Autodesk Inventor part; units mm, degrees
ref_plane "YZ Plane" through (0, 0, 0) normal (1, 0, 0) x (0, 1, 0)
ref_plane "XZ Plane" through (0, 0, 0) normal (0, 1, 0) x (-1, 0, 0)
ref_plane "XY Plane" through (0, 0, 0) normal (0, 0, 1) x (1, 0, 0)
sketch "Sketch1" plane through (0, 0, 0) normal (0, 1, 0) x (-1, 0, 0)
  line L0 (0, -3) -> (-10, -3)
  circle A0 centre (-21.6, 11.1) radius 1.5
  line L1 (0, 35) -> (-45, 35)
  line L2 (0, 0) -> (0, 35)
  circle A1 centre (-29.1, -17.1) radius 1.5
  arc A2 (-17.7344, 10.0719) -> (-25.4656, 12.1281) centre (-21.6, 11.1) ccw
  arc A3 (-32.9656, -16.0719) -> (-25.2344, -18.1281) centre (-29.1, -17.1) ccw
  line L3 (-17.7344, 10.0719) -> (-25.2344, -18.1281)
  line L4 (-27.4944, 4.5) -> (-35.4944, 4.5)
  line L5 (-35.4944, 4.5) -> (-35.4944, -10.5)
  line L6 (-35.4944, -10.5) -> (-31.4837, -10.5)
  line L7 (-25.4656, 12.1281) -> (-27.4944, 4.5)
  line L8 (-31.4837, -10.5) -> (-32.9656, -16.0719)
  point P0 (-35.4944, -3)
  dimension "d0" = 10
  dimension "d1" = 3
  dimension "d2" = 14.1
  dimension "d3" = 3
  dimension "d7" = 45
  dimension "d8" = 35
  dimension "d9" = 23.4
  dimension "d10" = 3
  dimension "d11" = 14.1
  dimension "d12" = 15.9
  dimension "d13" = 2.5
  dimension "d14" = 2.5
  dimension "d15" = 15
  dimension "d16" = 8
extrude "Extrusion1" add sketch "Sketch1" along normal blind 2.7
fillet "Fillet1" radius 2 4 edges at (35.4944, 1.35, 4.5) (27.4944, 1.35, 4.5) (35.4944, 1.35, -10.5) (31.4837, 1.35, -10.5)
properties part number "SujecionServo"
Input: part model. Units: mm. Frame: model coordinates. A direction names the side the tool comes from. Give positions to 0.01 mm unless a question says otherwise; leave off trailing zeros. Loops run counter-clockwise (first coordinate to the right, second up) from the corner with the lowest first, then second, coordinate; pieces in that order, holes last.
1) Section query B-B on z = 11.1. Return the cut outline in (x, y), and give its area (3 significant figures).
A:
outline: (17.6, 0) - (20.1, 0) - (20.1, 2.7) - (17.6, 2.7) - close; (23.1, 0) - (25.74, 0) - (25.74, 2.7) - (23.1, 2.7) - close
area: 13.9 mm2
2) Contact query for flat-ended pins moving along their axis: pin 1 (1.4 mm diameter, centred on x = 31.5, y = 1, fed in from +Z); pin 2 (1.5 mm diameter, centred on y = 1.5, z = -3, fed in from -X); pin 3 (8 mm diameter, centred on x = 33, z = 10.5, fed in from +Y). Output: stop coordinate, or through.
A:
pin 1: stops at z = 4.5
pin 2: stops at x = 21.01
pin 3: passes through
3) Section query C-C on y = 0.6. Count the separate pieces of the cut face and the enclosed holes in it, and give its area (3 significant figures).
A:
separate pieces: 1
enclosed holes: 2
area: 360 mm2
4) Mould query, pull axis X, two halves, no side actions, for faces 3 (the flat face through (32.548, 1.331, -14.5)), 4 (the flat face through (27, 0, -3)), 5 (the cylindrical face through (20.17, 1.33, 10.65)), 6 (the cylindrical face through (27.67, 1.33, -17.55)). Classes: released by +X, released by -X, zero draft, split by the parting line, or undercut.
A:
face 3: released by +X
face 4: zero draft
face 5: undercut
face 6: undercut
5) Section query A-A on x = 21.6. Return the cut outline in (y, z), and give its area (3 significant figures).
A:
outline: (0, -4.46) - (2.7, -4.46) - (2.7, 9.6) - (0, 9.6) - close; (0, 12.6) - (2.7, 12.6) - (2.7, 15.1) - (0, 15.1) - close
area: 44.7 mm2
6) Reachability of faces 1 (the flat face through (31, 1, 4.5)), 2 (the flat face through (27, 2.7, -3)) from +Z, -Z, +X, -X, +Y, -Y: full face, straight path, thin tool, end or side. Return the list, or none.
A:
face 1: +Z, +X, +Y, -Y
face 2: +Z, -Z, +X, -X, +Y
7) Section query D-D on x = 34.25. Return the cut outline in (y, z).
A:
outline: (0, -10.35) - (2.7, -10.35) - (2.7, 4.35) - (0, 4.35) - close
8) Line query: L1, parallel to Z at x = 29.1, y = 2.15; L2, parallel to X at y = 0.2, z = -12; L3, parallel to X at y = 0.35, z = -13. Output: solid intervals per line, ascending.
A:
L1: z = -21.1 to -18.6, -15.6 to 4.5
L2: x = 23.6 to 32.13
L3: x = 23.87 to 32.15
